Verification items for the finished model (mm, model axes). A direction names the side the tool comes from. Give positions to 0.01 mm unless a question says otherwise; leave off trailing zeros. Loops run counter-clockwise (first coordinate to the right, second up) from the corner with the lowest first, then second, coordinate; pieces in that order, holes last. Notation, with made-up numbers: (34.5, 39.25) -> (48.5, 39.25) arc R27 ccw to (48.5, 71.25) -> close; hole circle Ø4 at (62, -17). An arc over 180 degrees is marked (long way). Answer in a Markdown table with one row per item. Add a question column.
Q1. Section check D-D on y = 110. Enter the section's corners in (x, z).
Q2. Section check A-A on y = 11. Enter the section's corners in (x, z), and give its area (3 significant figures).
Q3. Section check C-C on x = 26. Enter the section's corners in (y, z), and give its area (3 significant figures).
Q4. Release check for a two-part mould opening along Y. For faces 4 (the face through (78, 100, 2)), 5 (the face through (74, 0, 1)), 6 (the face through (39, 76, 0)) record: pulls with the +Y half, pulls with the -Y half, needs draft (parallel to the pull), parting line crosses it, or undercut.
Q5. Gauge pin test, flat ends, axial feed: P1, Ø1.5, axis at x = 41, z = 1, coming from the -Y side; P2, Ø1.5, axis at y = 39, z = 1.5, coming from the -X side; P3, Ø1.5, axis at x = 1, z = 1, coming from the +Y side. Record the tip position at first contact, or that the pin passes through.
Q6. Material ranges on probe 1 along X at (y, z) = (26.5, 2.45); probe 2 along X at (y, z) = (54, 0.7); probe 3 along X at (y, z) = (89, 0.6), recorded low to high.
Q7. Set-up check for faces 1 (the face through (79, 50, 2)), 2 (the face through (62, 3, 2)), 3 (the face through (3, 25, 2)): record each of +Z, -Z, +X, -X, +Y, -Y from which the full face is reachable in a straight line by a thin tool's end or side.
Q8. Section check B-B on z = 2.4. Enter the section's corners in (x, y), and give its area (4 significant figures).
Autodesk Inventor part; units mm, degrees
ref_plane "YZ Plane" through (0, 0, 0) normal (1, 0, 0) x (0, 1, 0)
ref_plane "XZ Plane" through (0, 0, 0) normal (0, 1, 0) x (-1, 0, 0)
ref_plane "XY Plane" through (0, 0, 0) normal (0, 0, 1) x (1, 0, 0)
sketch "Boceto1" plane through (0, 0, 0) normal (0, 0, 1) x (1, 0, 0)
  line L0 (0, 0) -> (80, 0)
  line L1 (80, 0) -> (80, 150)
  line L2 (80, 150) -> (0, 150)
  line L3 (0, 150) -> (0, 0)
  dimension "d0" = 80
  dimension "d1" = 150
extrude "Extrusión1" add sketch "Boceto1" along normal blind 3
sketch "Boceto2" plane through (0, 0, 3) normal (0, 0, 1) x (1, 0, 0)
  line L0 (0, 0) -> (80, 0) construction
  line L1 (80, 0) -> (80, 150) construction
  line L2 (80, 150) -> (0, 150) construction
  line L3 (0, 150) -> (0, 0) construction
  line L4 (3, 0) -> (0, 0)
  line L5 (0, 0) -> (0, 50)
  line L6 (0, 50) -> (3, 50)
  line L7 (3, 50) -> (3, 0)
  line L8 (0, 150) -> (3, 150)
  line L9 (3, 150) -> (3, 100)
  line L10 (3, 100) -> (0, 100)
  line L11 (0, 100) -> (0, 150)
  line L12 (77, 100) -> (80, 100)
  line L13 (80, 100) -> (80, 50)
  line L14 (80, 50) -> (77, 50)
  line L15 (77, 50) -> (77, 100)
  line L16 (80, 0) -> (80, 150) construction
  point P0 (80, 75)
  point P1 (80, 75)
  dimension "d4" = 3
  dimension "d5" = 50
  dimension "d6" = 3
  dimension "d7" = 50
  dimension "d8" = 50
  dimension "d9" = 3
extrude "Extrusión2" cut sketch "Boceto2" against normal blind 3
sketch "Boceto3" plane through (0, 0, 3) normal (0, 0, 1) x (1, 0, 0)
  line L0 (3, 50) -> (3, 0) construction
  line L1 (3, 0) -> (80, 0) construction
  line L2 (80, 0) -> (80, 50) construction
  line L3 (80, 50) -> (77, 50) construction
  line L4 (77, 50) -> (77, 100) construction
  line L5 (77, 100) -> (80, 100) construction
  line L6 (80, 100) -> (80, 150) construction
  line L7 (80, 150) -> (3, 150) construction
  line L8 (3, 150) -> (3, 100) construction
  line L9 (3, 100) -> (0, 100) construction
  line L10 (0, 100) -> (0, 50) construction
  line L11 (0, 50) -> (3, 50) construction
  line L12 (40, 70) -> (43, 70)
  line L13 (43, 70) -> (43, 0)
  line L14 (43, 0) -> (40, 0)
  line L15 (40, 0) -> (40, 70)
  line L16 (3, 0) -> (80, 0) construction
  point P0 (0, 0)
  point P1 (41.5, 0)
  point P2 (41.5, 0)
  dimension "d12" = 3
  dimension "d13" = 70
extrude "Extrusión3" cut sketch "Boceto3" against normal blind 10
sketch "Boceto4" plane through (0, 0, 3) normal (0, 0, 1) x (1, 0, 0)
  line L0 (43, 70) -> (43, 0) construction
  line L1 (43, 0) -> (80, 0) construction
  line L2 (80, 0) -> (80, 50) construction
  line L3 (80, 50) -> (77, 50) construction
  line L4 (77, 50) -> (77, 100) construction
  line L5 (77, 100) -> (80, 100) construction
  line L6 (80, 100) -> (80, 150) construction
  line L7 (80, 150) -> (3, 150) construction
  line L8 (3, 150) -> (3, 100) construction
  line L9 (3, 100) -> (0, 100) construction
  line L10 (0, 100) -> (0, 50) construction
  line L11 (0, 50) -> (3, 50) construction
  line L12 (3, 50) -> (3, 0) construction
  line L13 (3, 0) -> (40, 0) construction
  line L14 (40, 0) -> (40, 70) construction
  line L15 (40, 70) -> (43, 70) construction
  line L16 (14, 3) -> (29, 3)
  line L17 (29, 3) -> (29, 0)
  line L18 (29, 0) -> (14, 0)
  line L19 (14, 0) -> (14, 3)
  line L20 (69, 3) -> (54, 3)
  line L21 (54, 3) -> (54, 0)
  line L22 (54, 0) -> (69, 0)
  line L23 (69, 0) -> (69, 3)
  line L24 (3, 0) -> (40, 0) construction
  point P0 (0, 0)
  point P1 (61.5, 0)
  point P2 (61.5, 0)
  point P3 (21.5, 0)
  point P4 (21.5, 0)
  dimension "d16" = 3
  dimension "d17" = 3
  dimension "d18" = 15
  dimension "d19" = 15
extrude "Extrusión4" cut sketch "Boceto4" against normal blind 10
equation "\"d6\" = d4"
equation "\"d7\" = d5"
equation "\"d8\" = d7"
equation "\"d9\" = d4"
equation "\"d19\" = d18"
properties part number "Pared Garita2"
Taken from the geometry:
| question | item | result |
|---|---|---|
| 1 | outline | (3, 0) -> (80, 0) -> (80, 3) -> (3, 3) -> close |
| 2 | outline | (3, 0) -> (40, 0) -> (40, 3) -> (3, 3) -> close; (43, 0) -> (80, 0) -> (80, 3) -> (43, 3) -> close |
| 2 | area | 222 mm² |
| 3 | outline | (3, 0) -> (150, 0) -> (150, 3) -> (3, 3) -> close |
| 3 | area | 441 mm² |
| 4 | face 4 | undercut |
| 4 | face 5 | pulls with the -Y half |
| 4 | face 6 | needs draft |
| 5 | P1 | stops at y = 70 |
| 5 | P2 | stops at x = 3 |
| 5 | P3 | stops at y = 100 |
| 6 | probe 1 | x = 3 to 40, 43 to 80 |
| 6 | probe 2 | x = 0 to 40, 43 to 77 |
| 6 | probe 3 | x = 0 to 77 |
| 7 | face 1 | +Z, -Z, +X |
| 7 | face 2 | +Z, -Z, -Y |
| 7 | face 3 | +Z, -Z, -X, -Y |
| 8 | outline | (0, 50) -> (3, 50) -> (3, 0) -> (14, 0) -> (14, 3) -> (29, 3) -> (29, 0) -> (40, 0) -> (40, 70) -> (43, 70) -> (43, 0) -> (54, 0) -> (54, 3) -> (69, 3) -> (69, 0) -> (80, 0) -> (80, 50) -> (77, 50) -> (77, 100) -> (80, 100) -> (80, 150) -> (3, 150) -> (3, 100) -> (0, 100) -> close |
| 8 | area | 11,250 mm² |
